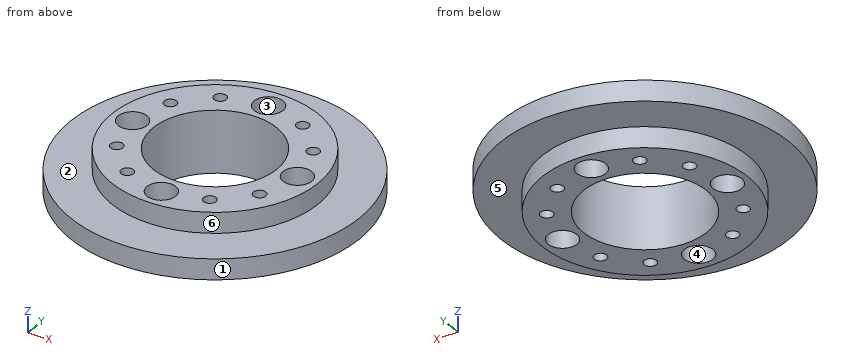
```python
from build123d import *

# Parameters (mm, degrees)
SKETCH1_R               = 12.5
BOSS_EXTRUDE1_DEPTH     = 2.5
SKETCH3_R               = 17.5
BOSS_EXTRUDE2_DEPTH     = 2.5
BOSS_EXTRUDE3_START     = 2.5
SKETCH5_R               = 12.5
BOSS_EXTRUDE3_DEPTH     = 2.5
CUT_EXTRUDE1_DEPTH      = 26.860201082
CUT_EXTRUDE1_DEPTH_BACK = 26.860201082
SKETCH2_R               = 0.75
SKETCH2_R_2             = 7.5
SKETCH6_R               = 1.75
CUT_EXTRUDE2_DEPTH      = 10


with BuildPart() as part:
    # Sketch1 → Boss-Extrude1 (new body)
    with BuildSketch(Plane.XY):
        Circle(SKETCH1_R)
    extrude(amount=BOSS_EXTRUDE1_DEPTH)

    # Sketch3 → Boss-Extrude2 (add)
    with BuildSketch(Plane(origin=(0, 0, 0), x_dir=(-1, 0, 0), z_dir=(0, 0, -1))):
        Circle(SKETCH3_R)
    extrude(amount=BOSS_EXTRUDE2_DEPTH)

    # Sketch5 → Boss-Extrude3 (add)
    with BuildSketch(Plane(origin=(0, 0, -2.5), x_dir=(-1, 0, 0), z_dir=(0, 0, -1)).offset(BOSS_EXTRUDE3_START)):
        with Locations(Location((0, 0, 0), (0, 0, 180))):
            Circle(SKETCH5_R)
    extrude(amount=-BOSS_EXTRUDE3_DEPTH)

    # Sketch2 → Cut-Extrude1 (cut, two sides: drawn at the far end of the back side and taken through both)
    with BuildSketch(Plane.XY.offset(2.5).offset(-CUT_EXTRUDE1_DEPTH_BACK)):
        with Locations((0, 10)):
            Circle(SKETCH2_R)
        with Locations((5, 8.660254038)):
            Circle(SKETCH2_R)
        with Locations((8.660254038, 5)):
            Circle(SKETCH2_R)
        with Locations((10, 0)):
            Circle(SKETCH2_R)
        with Locations((8.660254038, -5)):
            Circle(SKETCH2_R)
        with Locations((5, -8.660254038)):
            Circle(SKETCH2_R)
        with Locations((0, -10)):
            Circle(SKETCH2_R)
        with Locations((-5, -8.660254038)):
            Circle(SKETCH2_R)
        with Locations((-8.660254038, -5)):
            Circle(SKETCH2_R)
        with Locations((-10, 0)):
            Circle(SKETCH2_R)
        with Locations((-8.660254038, 5)):
            Circle(SKETCH2_R)
        with Locations((-5, 8.660254038)):
            Circle(SKETCH2_R)
        Circle(SKETCH2_R_2)
    extrude(amount=CUT_EXTRUDE1_DEPTH + CUT_EXTRUDE1_DEPTH_BACK, mode=Mode.SUBTRACT)

    # Sketch6 → Cut-Extrude2 (cut)
    with BuildSketch(Plane(origin=(0, 0, -5), x_dir=(-1, 0, 0), z_dir=(0, 0, -1))):
        with Locations((0, 10)):
            Circle(SKETCH6_R)
        with Locations((10, 0)):
            Circle(SKETCH6_R)
        with Locations((0, -10)):
            Circle(SKETCH6_R)
        with Locations((-10, 0)):
            Circle(SKETCH6_R)
    extrude(amount=-CUT_EXTRUDE2_DEPTH, mode=Mode.SUBTRACT)


solid = part.part
```
Input: part model. Units: mm. Frame: model coordinates. Face numbers are marked on the shaded views. A direction names the side the tool comes from. Give positions to 0.01 mm unless a question says otherwise; leave off trailing zeros. Order: outer loops, then holes, each group sorted by start corner. A loop starts at its lowest first (then second) coordinate and runs counter-clockwise, first axis right, second up. Notation, with made-up numbers: M 31,37.5 L 67,37.5 A26 cw 67,67.5 Z; hole C 46,-10 d6. An arc over 180 degrees is marked long. Return JSON: item names as keys, results as strings.
1) Mould query, pull axis X, two halves, no side actions, for the marked faces 1, 2 and 3. Classes: released by +X, released by -X, zero draft, split by the parting line, or undercut.
Taken from the geometry:
{"face 1": "split by the parting line", "face 2": "zero draft", "face 3": "undercut"}
2) Section query C-C on z = -0.5. Count the separate pieces of the cut face and the enclosed holes in it, and give its area (3 significant figures).
Taken from the geometry:
{"separate pieces": "1", "enclosed holes": "13", "area": "733 mm2"}
3) Line query: L1, parallel to Y at x = 10, z = -4; L2, parallel to X at y = -1.5, z = -0.5; L3, parallel to Y at x = -4.5, z = -0.5. Output: solid intervals per line, ascending. Write a range as [from, to].
Taken from the geometry:
{"L1": "y = [-7.5, -1.75], [1.75, 7.5]", "L2": "x = [-17.44, -10.9], [-9.1, -7.35], [7.35, 9.1], [10.9, 17.44]", "L3": "y = [-16.91, -9.22], [-8.1, -6], [6, 8.1], [9.22, 16.91]"}
4) Section query D-D on x = 10. Output: boundary loops of the cut face in (y, z), and give its area (3 significant figures).
Taken from the geometry:
{"outline": "M -14.36,-2.5 L -7.5,-2.5 L -7.5,-5 L -1.75,-5 L -1.75,2.5 L -7.5,2.5 L -7.5,0 L -14.36,0 Z; M 1.75,-5 L 7.5,-5 L 7.5,-2.5 L 14.36,-2.5 L 14.36,0 L 7.5,0 L 7.5,2.5 L 1.75,2.5 Z", "area": "121 mm2"}
5) Access query for the marked faces 4, 5 and 6. Directions: +Z, -Z, +X, -X, +Y, -Y. A direction counts if a zero-diameter tool reaches every point of the face in a straight line with its end or side. Return the directions, or none.
Taken from the geometry:
{"face 4": "+Z, -Z", "face 5": "-Z", "face 6": "+Z"}
6) Contact query for flat-ended pins moving along their axis: pin 1 (2 mm diameter, centred on y = 6, z = -1, fed in from -X); pin 2 (3 mm diameter, centred on x = -12, z = -1.5, fed in from +Y); pin 3 (1 mm diameter, centred on x = -12, y = -9, fed in from +Z). Output: stop coordinate, or through.
Taken from the geometry:
{"pin 1": "stops at x = -16.77", "pin 2": "stops at y = 14", "pin 3": "stops at z = 0"}
7) Section query A-A on x = 0. Output: boundary loops of the cut face in (y, z).
Taken from the geometry:
{"outline": "M -17.5,-2.5 L -12.5,-2.5 L -12.5,-5 L -11.75,-5 L -11.75,2.5 L -12.5,2.5 L -12.5,0 L -17.5,0 Z; M -8.25,-5 L -7.5,-5 L -7.5,2.5 L -8.25,2.5 Z; M 7.5,-5 L 8.25,-5 L 8.25,2.5 L 7.5,2.5 Z; M 11.75,-5 L 12.5,-5 L 12.5,-2.5 L 17.5,-2.5 L 17.5,0 L 12.5,0 L 12.5,2.5 L 11.75,2.5 Z"}
